Part model, mm, in its own coordinate system. Face numbers are marked on the shaded views. A direction names the side the tool comes from. Give positions to 0.01 mm unless a question says otherwise; leave off trailing zeros. Order: outer loops, then holes, each group sorted by start corner. A loop starts at its lowest first (then second) coordinate and runs counter-clockwise, first axis right, second up. Notation, with made-up numbers: (79, 60) -> (91, 60) arc R11 cw to (91, 69) -> close; hole circle Ø9 at (-38, 82). An arc over 180 degrees is marked (long way). Write item = value, one per line. Start each with the question number.
Item 1: Band-saw the part on C-C on x = -179. Write the cut outline in (y, z), plus the area to 3 significant figures.
Item 2: Band-saw the part on B-B on z = 120. Write the cut outline in (x, y), plus the area to 3 significant figures.
Item 3: Flat gauge pins, fed straight in: P1, Ø4, axis at x = 29.5, z = 1, coming from the -Y side; P2, Ø7.5, axis at x = -27, z = -1.5, coming from the -Y side; P3, Ø6, axis at x = -130.5, z = 150, coming from the -Y side; P4, Ø9, axis at y = -71.5, z = 115, coming from the +X side. Where does each tip first touch, or does it go through?
Item 4: Pull direction Z, two halves, no side cores. Call the marked faces 4, 5 and 6: +Z half, -Z half, draft (parallel to the pull), parting line (faces both ways), or undercut.
Item 5: Drill centre lines: line 1 along X through (y, z) = (-83.1, 0); line 2 along Y through (x, z) = (-40, 131.5); line 3 along Z through (x, y) = (30, -81.5). Where is each one in solid material? Low to high.
Item 6: Band-saw the part on D-D on y = 11.5. Write the cut outline in (x, z).
Item 7: Band-saw the part on A-A on y = -44. Count the separate pieces of the cut face and the enclosed holes in it, plus the area to 3 significant figures.
Item 8: Tool access for the marked faces 1, 2 and 3: list every direction of +Z, -Z, +X, -X, +Y, -Y with a clear straight run to the whole face (end or side of a thin tool).
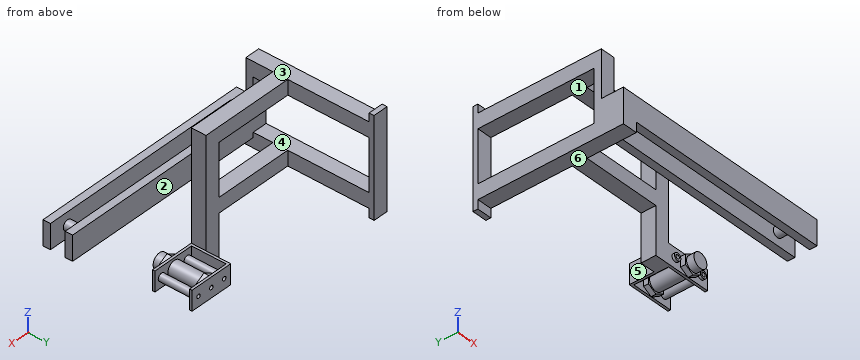
```python
from build123d import *

# Parameters (mm, degrees)
F0_W      = 90
F0_H      = 40
F0_R      = 4
F1_DEPTH  = 5
F3_DEPTH  = 10
F4_R      = 15
F5_DEPTH  = 60
F6_R      = 7.5
F6_R_2    = 4
F7_DEPTH  = 80
F8_W      = 90
F8_H      = 40
F9_DEPTH  = 5
F11_DEPTH = 10
F12_R     = 15
F13_DEPTH = 15
F14_W     = 5
F14_H     = 40
F15_DEPTH = 70
F16_R     = 4
F17_DEPTH = 50
F18_W     = 30
F18_H     = 260
F19_DEPTH = 30
F20_W     = 30
F20_H     = 30
F21_DEPTH = 190
F22_W     = 30
F22_H     = 30
F23_DEPTH = 205
F24_DEPTH = 40
F25_W     = 30
F25_H     = 200
F26_DEPTH = 10
F27_W     = 30
F27_H     = 165
F28_DEPTH = 60
F29_W     = 15
F29_H     = 50
F30_DEPTH = 420
F31_W     = 45
F31_H     = 121.339908
F32_DEPTH = 40
F33_R     = 10
F34_DEPTH = 60


with BuildPart() as f1:
    # F0 (on Front) → F1 (new body)
    with BuildSketch(Plane.XZ):
        Rectangle(F0_W, F0_H)
        with Locations((-30, 0)):
            Circle(F0_R, mode=Mode.SUBTRACT)
        Circle(F0_R, mode=Mode.SUBTRACT)
        with Locations((30, 0)):
            Circle(F0_R, mode=Mode.SUBTRACT)
    extrude(amount=F1_DEPTH)

    # F2 (on face) → F3 (join)
    with BuildSketch(Plane.XZ.offset(5)):
        Polygon((17.5, -10.10363), (17.5, 10.10363), (0, 20.207259), (-17.5, 10.10363), (-17.5, -10.10363), (0, -20.207259), align=None)
    extrude(amount=F3_DEPTH)

    # F4 (on face) → F5 (join)
    with BuildSketch(Plane.XZ.offset(15)):
        Circle(F4_R)
    extrude(amount=F5_DEPTH)

    # F6 (on face) → F7 (join)
    with BuildSketch(Plane.XZ.offset(5)):
        with Locations((30, 0)):
            Circle(F6_R)
        with Locations((30, 0)):
            Circle(F6_R_2, mode=Mode.SUBTRACT)
        with Locations((-30, 0)):
            Circle(F6_R)
        with Locations((-30, 0)):
            Circle(F6_R_2, mode=Mode.SUBTRACT)
    extrude(amount=F7_DEPTH)

    # F8 (on face) → F9 (join)
    with BuildSketch(Plane.XZ.offset(75)):
        Rectangle(F8_W, F8_H)
    extrude(amount=F9_DEPTH)

    # F10 (on face) → F11 (join)
    with BuildSketch(Plane.XZ.offset(80)):
        Polygon((0.040823, -20.207218), (17.520376, -10.068255), (17.479553, 10.138963), (-0.040823, 20.207218), (-17.520376, 10.068255), (-17.479553, -10.138963), align=None)
    extrude(amount=F11_DEPTH)

    # F12 (on face) → F13 (join)
    with BuildSketch(Plane.XZ.offset(90)):
        Circle(F12_R)
    extrude(amount=F13_DEPTH)

    # F14 (on face) → F15 (join, through all)
    with BuildSketch(Plane.XZ.offset(5)):
        with Locations((-42.5, 0)):
            Rectangle(F14_W, F14_H)
    extrude(amount=F15_DEPTH)

    # F16 (on face) → F17 (cut)
    with BuildSketch(Plane(origin=(0, 0, 0), x_dir=(-1, 0, 0), z_dir=(0, 1, 0))):
        Circle(F16_R)
    extrude(amount=-F17_DEPTH, mode=Mode.SUBTRACT)

    # F18 (on face) → F19 (join)
    with BuildSketch(Plane(origin=(-45, 0, 0), x_dir=(0, -1, 0), z_dir=(-1, 0, 0))):
        with Locations((65, 110)):
            Rectangle(F18_W, F18_H)
    extrude(amount=F19_DEPTH)

    # F20 (on face) → F21 (join)
    with BuildSketch(Plane(origin=(-75, 0, 0), x_dir=(0, -1, 0), z_dir=(-1, 0, 0))):
        with Locations((65, 90)):
            Rectangle(F20_W, F20_H)
        with Locations((65, 225)):
            Rectangle(F20_W, F20_H)
    extrude(amount=F21_DEPTH)

    # F22 (on face) → F23 (join)
    with BuildSketch(Plane.XZ.offset(80)):
        with Locations((-250, 90)):
            Rectangle(F22_W, F22_H)
        with Locations((-250, 225)):
            Rectangle(F22_W, F22_H)
    extrude(amount=-F23_DEPTH)

    # F22 (on face) → F24 (join)
    with BuildSketch(Plane.XZ.offset(80)):
        with Locations((-250, 90)):
            Rectangle(F22_W, F22_H)
        with Locations((-250, 225)):
            Rectangle(F22_W, F22_H)
    extrude(amount=F24_DEPTH)

    # F25 (on face) → F26 (join)
    with BuildSketch(Plane(origin=(0, 125, 0), x_dir=(-1, 0, 0), z_dir=(0, 1, 0))):
        with Locations((250, 157)):
            Rectangle(F25_W, F25_H)
    extrude(amount=-F26_DEPTH)

    # F27 (on face) → F28 (join)
    with BuildSketch(Plane.XZ.offset(120)):
        with Locations((-250, 157.5)):
            Rectangle(F27_W, F27_H)
    extrude(amount=F28_DEPTH)

    # F29 (on face) → F30 (join)
    with BuildSketch(Plane.YZ.offset(-235)):
        with Locations((-172.5, 120)):
            Rectangle(F29_W, F29_H)
        with Locations((-127.5, 120)):
            Rectangle(F29_W, F29_H)
    extrude(amount=F30_DEPTH)

    # F31 (on face) → F32 (cut)
    with BuildSketch(Plane.YZ.offset(-235)):
        with Locations((-157.5, 205.669954)):
            Rectangle(F31_W, F31_H)
    extrude(amount=-F32_DEPTH, mode=Mode.SUBTRACT)

    # F33 (on face) → F34 (join)
    with BuildSketch(Plane.XZ.offset(180)):
        with Locations((145, 120)):
            Circle(F33_R)
    extrude(amount=-F34_DEPTH)


solid = f1.part
```
Values found:
q1.outline = (-180, 95) -> (-165, 95) -> (-165, 145) -> (-180, 145) -> close; (-135, 95) -> (-120, 95) -> (-120, 145) -> (-135, 145) -> close; (-80, 75) -> (-50, 75) -> (-50, 105) -> (-80, 105) -> close; (-80, 210) -> (-50, 210) -> (-50, 240) -> (-80, 240) -> close
q1.area = 3,300 mm^2
q2.outline = (-265, -180) -> (185, -180) -> (185, -165) -> (155, -165) -> (155, -135) -> (185, -135) -> (185, -120) -> (-265, -120) -> close; (-265, 115) -> (-235, 115) -> (-235, 125) -> (-265, 125) -> close; (-75, -80) -> (-45, -80) -> (-45, -50) -> (-75, -50) -> close; hole (-235, -165) -> (135, -165) -> (135, -135) -> (-235, -135) -> close
q2.area = 16,200 mm^2
q3.P1 = -80
q3.P2 = -85
q3.P3 = through
q3.P4 = -45
q4.face_4 = undercut
q4.face_5 = draft
q4.face_6 = -Z half
q5.line_1 = -37.5 to -34, -26 to -22.5, -17.5 to 17.5, 22.5 to 26, 34 to 37.5
q5.line_2 = -180 to -165, -135 to -120
q5.line_3 = -7.5 to -4, 4 to 7.5
q6.outline = (-265, 75) -> (-235, 75) -> (-235, 105) -> (-265, 105) -> close; (-265, 210) -> (-235, 210) -> (-235, 240) -> (-265, 240) -> close
q7.separate_pieces = 6
q7.enclosed_holes = 3
q7.area = 2,910 mm^2
q8.face_1 = -X
q8.face_2 = +X
q8.face_3 = +Z, +X, -X, -Y
